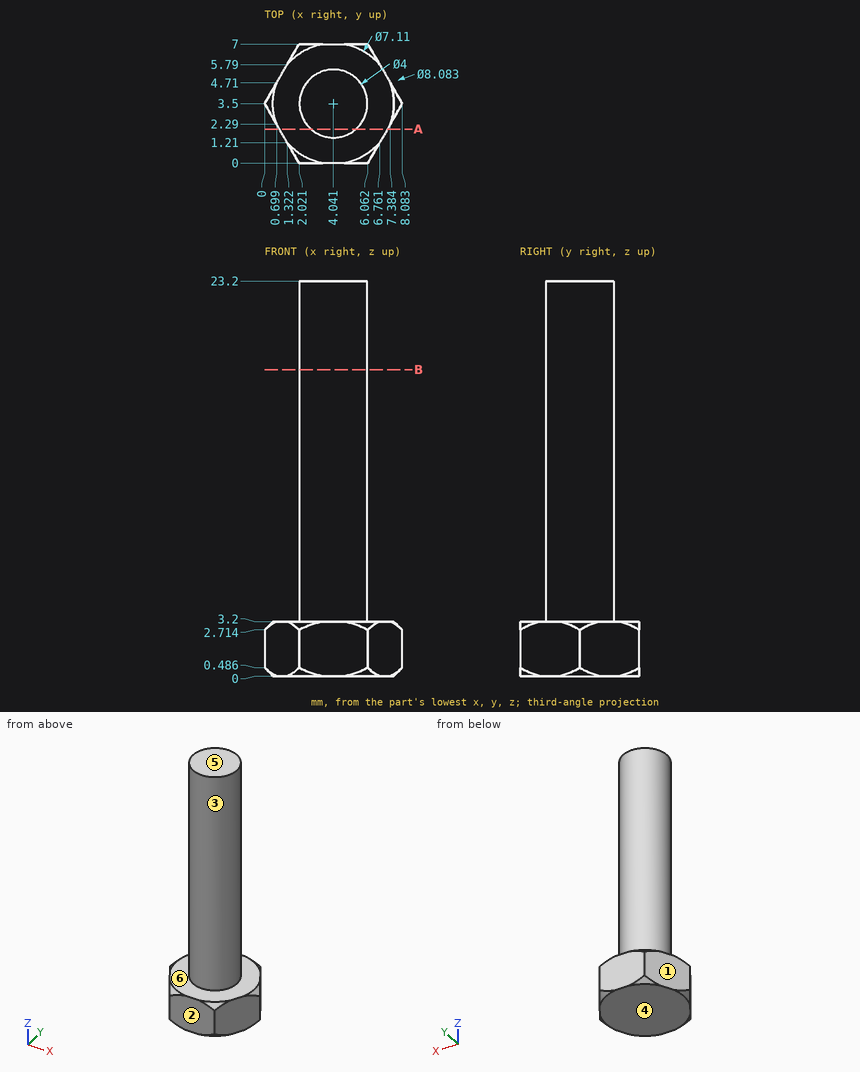
Verification items for this drawing (mm, ordinates from the low corner). A direction names the side the tool comes from. Coordinates: 2 decimals unless noted, no trailing zeros. Order: outer loops, then holes, each group sorted by start corner. A loop starts at its lowest first (then second) coordinate and runs counter-clockwise, first axis right, second up. Notation, with made-up numbers: M 71.25,34 L 125.25,34 A27 ccw 125.25,71 Z; hole C 67,83 d2. An arc over 180 degrees is marked long. Answer as a JSON object with one key per item and string values.
Q1. Cross-section at A-A on y = 2. Record the cut outline in (x, z) (1 decimal).
Results are:
{"outline": "M 0.9,0 L 7.2,0 L 7.2,3.2 L 5.4,3.2 L 5.4,23.2 L 2.7,23.2 L 2.7,3.2 L 0.9,3.2 Z"}
Q2. Scan lines: line 1 (Z direction, x = 2.5, y = 1.5); line 2 (Y direction, x = 1.25, z = 2.25) (1 decimal); line 3 (X direction, y = 2, z = 13.5) (1 decimal). Record each from-to range of solid material in increasing order.
Results are:
{"line 1": "z = 0 to 3.2", "line 2": "y = 1.3 to 5.7", "line 3": "x = 2.7 to 5.4"}
Q3. Tool access check on the marked faces 5 and 6. Record the directions out of +Z, -Z, +X, -X, +Y, -Y that give a thin tool (end or side, any length) a straight path to the whole face; none if there is none.
Results are:
{"face 5": "+Z, +X, -X, +Y, -Y", "face 6": "+Z"}
Q4. Release check for a two-part mould opening along Y. For the marked faces 1, 2, 3 and 4 record: released by +Y, released by -Y, zero draft, split by the parting line, or undercut.
Results are:
{"face 1": "released by +Y", "face 2": "released by -Y", "face 3": "split by the parting line", "face 4": "zero draft"}
Q5. Depth check by flat-ended pin: pin 1 Ø2 at (x, z) = (4.5, 7) entering from +Y; pin 2 Ø1.5 at (y, z) = (2, 18) entering from +X (1 decimal); pin 3 Ø1 at (x, z) = (5, 10) entering from +Y. Enter the tip coordinate at first touch or a pass-through.
Results are:
{"pin 1": "stops at y = 5.5", "pin 2": "stops at x = 5.9", "pin 3": "stops at y = 5.45"}
Q6. Cross-section at B-B on z = 18. Record the cut outline in (x, y), and give its area (3 significant figures).
Results are:
{"outline": "C 4.04,3.5 d4", "area": "12.6 mm²"}
